```python
from build123d import *

# Parameters (mm, degrees)
F0_W     = 6
F0_H     = 8
F0_W_2   = 24
F1_DEPTH = 3
F2_D     = 2.9
F4_D     = 2.3
F5_R     = 1


with BuildPart() as f1:
    # F0 (on Top) → F1 (new body)
    with BuildSketch(Plane.XY):
        Rectangle(F0_W, F0_H)
        with Locations((15, 0)):
            Rectangle(F0_W_2, F0_H)
        with Locations((30, 0)):
            Rectangle(F0_W, F0_H)
    extrude(amount=-F1_DEPTH)

    # F2 (through all)
    with Locations(Plane.XY):
        with Locations((0, 0), (4, 0), (26, 0), (30, 0)):
            Hole(F2_D / 2)

    # F4 (through all)
    with Locations(Plane.XZ.offset(4)):
        with Locations((9, 0), (21, 0), (15, 0)):
            Hole(F4_D / 2)

    # F5
    f5_edges = [f1.edges().sort_by_distance(p)[0] for p in [
        (-3, -4, -1.5),
        (33, -4, -1.5),
        (33, 4, -1.5),
        (-3, 4, -1.5),
    ]]
    fillet(f5_edges, radius=F5_R)


solid = f1.part
```
Design review of the part built by this model. Coordinates are the model's own, in mm. Give positions to 0.01 mm unless a question says otherwise; leave off trailing zeros. Write each loop counter-clockwise with the first axis right and the second up, starting at its lowest first coordinate (ties: lowest second). Pieces come first, ordered by that corner, then holes. Notation, with made-up numbers: (81.5, 39) - (128.5, 39) arc R18 cw to (128.5, 46) - close; hole circle Ø5 at (40, 28.25). An arc over 180 degrees is marked (long way). Return JSON: item names as keys, results as strings. Group by question number.
(1) To check wall thickness, follow probe 1 along X at (y, z) = (2.5, -0.6); probe 2 along Y at (x, z) = (0, -1); probe 3 along Y at (x, z) = (3, -0.45). State the ranges of each line that lie inside material, in increasing order.
(2) We need section B-B, the plane x = 26. Give the boundary of the cut face in (y, z).
(3) We need section C-C, the plane y = -0.75. Give the boundary of the cut face in (x, z).
(4) Insertion check: pin 1 (4 mm diameter, centred on x = 22, y = 2, fed in from +Z). The pin has a flat end and moves straight along its axis. Give the tip position at first contact, or say it passes through.
(5) We need section D-D, the plane z = -0.6. Give the boundary of the cut face in (x, y), then the cut area to 3 significant figures.
(6) Mouldability with a two-part tool opening along X and no side actions: class faces 1 (the cylindrical face through (32.699, 3.715, -1.521)), 2 (the cylindrical face through (9.03, 0.06, -1.15)), 3 (the flat face through (14.8, -4, -1.5)) as +X half, -X half, draft (parallel to the pull), parting line (faces both ways), or undercut.
(7) We need section A-A, the plane z = -2.1. Give the boundary of the cut face in (x, y).
Reported:
{
 "1": {"probe 1": "x = -3 to 8.02, 9.98 to 14.02, 15.98 to 20.02, 21.98 to 33", "probe 2": "y = -4 to -1.45, 1.45 to 4", "probe 3": "y = -4 to -1.05, 1.05 to 4"},
 "2": {"outline": "(-4, -3) - (-1.45, -3) - (-1.45, 0) - (-4, 0) - close; (1.45, -3) - (4, -3) - (4, 0) - (1.45, 0) - close"},
 "3": {"outline": "(-3, -3) - (-1.24, -3) - (-1.24, 0) - (-3, 0) - close; (1.24, -3) - (2.76, -3) - (2.76, 0) - (1.24, 0) - close; (5.24, -3) - (24.76, -3) - (24.76, 0) - (22.15, 0) arc R1.15 cw to (19.85, 0) - (16.15, 0) arc R1.15 cw to (13.85, 0) - (10.15, 0) arc R1.15 cw to (7.85, 0) - (5.24, 0) - close; (27.24, -3) - (28.76, -3) - (28.76, 0) - (27.24, 0) - close; (31.24, -3) - (33, -3) - (33, 0) - (31.24, 0) - close"},
 "4": {"pin 1": "stops at z = 0"},
 "5": {"outline": "(-3, -3) arc R1 ccw to (-2, -4) - (8.02, -4) - (8.02, 4) - (-2, 4) arc R1 ccw to (-3, 3) - close; (9.98, -4) - (14.02, -4) - (14.02, 4) - (9.98, 4) - close; (15.98, -4) - (20.02, -4) - (20.02, 4) - (15.98, 4) - close; (21.98, -4) - (32, -4) arc R1 ccw to (33, -3) - (33, 3) arc R1 ccw to (32, 4) - (21.98, 4) - close; hole circle Ø2.9 at (0, 0); hole circle Ø2.9 at (4, 0); hole circle Ø2.9 at (26, 0); hole circle Ø2.9 at (30, 0)", "area": "214 mm2"},
 "6": {"face 1": "+X half", "face 2": "undercut", "face 3": "draft"},
 "7": {"outline": "(-3, -3) arc R1 ccw to (-2, -4) - (32, -4) arc R1 ccw to (33, -3) - (33, 3) arc R1 ccw to (32, 4) - (-2, 4) arc R1 ccw to (-3, 3) - close; hole circle Ø2.9 at (0, 0); hole circle Ø2.9 at (4, 0); hole circle Ø2.9 at (26, 0); hole circle Ø2.9 at (30, 0)"}
}
